Read the model definition and answer for the solid it produces. Units are mm, in the model's axes. Give positions to 0.01 mm unless a question says otherwise; leave off trailing zeros. Write each loop counter-clockwise with the first axis right and the second up, starting at its lowest first coordinate (ties: lowest second). Pieces come first, ordered by that corner, then holes. Notation, with made-up numbers: (73, 67) -> (112, 67) arc R25 cw to (112, 84) -> close; hole circle Ø8 at (60.25, -1). An arc over 180 degrees is marked (long way). Put each result on its own line as item: value. Start each with the question number.
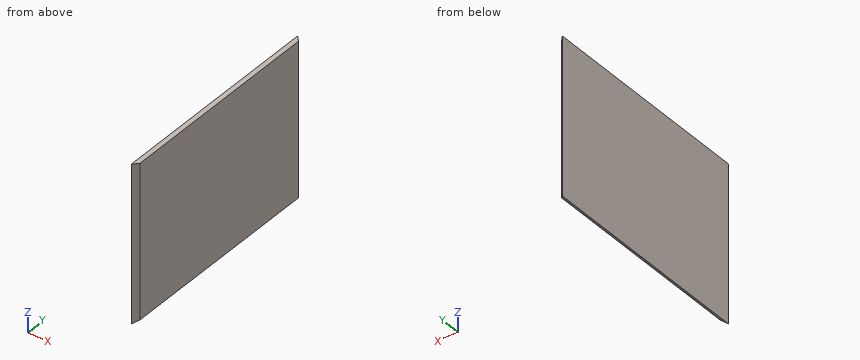
from build123d import *

# Parameters (mm, degrees)
F0_W     = 400
F0_H     = 300
F1_DEPTH = 9
F3_DEPTH = 300
F5_DEPTH = 400
F6_DEPTH = 30


# Not quite as in the source:
# - a feature names something its author has since deleted; it is built from what else it names


with BuildPart() as f1:
    # F0 (on Right) → F1 (new body)
    with BuildSketch(Plane.YZ):
        with Locations((176.1937195063, 136.9389362159)):
            Rectangle(F0_W, F0_H)
    extrude(amount=F1_DEPTH)

    # F2 (on face) → F3 (cut)
    with BuildSketch(Plane.XY.offset(286.9389362159)):
        Polygon((9, 376.1937195063), (0, 376.1937195063), (9, 367.1937195063), align=None)
        Polygon((9, -14.8062804937), (0, -23.8062804937), (9, -23.8062804937), align=None)
    extrude(amount=-F3_DEPTH, mode=Mode.SUBTRACT)

    # F4 (on Front) → F5 (cut)
    with BuildSketch(Plane.XZ):
        Polygon((9, -6.68870858), (0, -13.0610637841), (9, -13.0610637841), align=None)
    extrude(amount=-F5_DEPTH, mode=Mode.SUBTRACT)

    # F4 (on Front) → F6 (cut)
    with BuildSketch(Plane.XZ):
        Polygon((9, -6.68870858), (0, -13.0610637841), (9, -13.0610637841), align=None)
    extrude(amount=F6_DEPTH, mode=Mode.SUBTRACT)


solid = f1.part
1) A cutting plane is placed at A-A on z = 183. Give the vertices of the cut face in (x, y), and give its area (3 significant figures).
2) A cutting plane is placed at B-B on x = 5.75. Give the vertices of the cut face in (y, z), and give its area (3 significant figures).
3) Each of these flat-tipped pins is pushed along its axis until it touches: pin 1 Ø2 at (x, z) = (5, 133.5) entering from +Y; pin 2 Ø5 at (x, y) = (3, 33.5) entering from -Z. Where does it stop, or does it pass through?
4) Straight lines are drawn through the part: line 1 (Z direction, x = 3.75, y = 281.5); line 2 (Z direction, x = 3.5, y = 56.5); line 3 (Y direction, x = 4, z = 202.5). For each, find the intervals that lie inside material, in ascending order. Write a range as [from, to].
Results found:
1. outline: (0, -23.81) -> (9, -14.81) -> (9, 367.19) -> (0, 376.19) -> close
1. area: 3,520 mm²
2. outline: (-18.06, -8.99) -> (370.44, -8.99) -> (370.44, 286.94) -> (-18.06, 286.94) -> close
2. area: 115,000 mm²
3. pin 1: stops at y = 372.19
3. pin 2: stops at z = -12.71
4. line 1: z = [-10.41, 286.94]
4. line 2: z = [-10.58, 286.94]
4. line 3: y = [-19.81, 372.19]
